```python
from build123d import *

# Parameters (mm, degrees)
IZIM1_R                     = 5
Y_KSEKLIK_EKSTR_ZYON1_DEPTH = 15
IZIM2_R                     = 7.5
Y_KSEKLIK_EKSTR_ZYON2_DEPTH = 5
RADYUS1_R                   = 5
Y_KSEKLIK_EKSTR_ZYON3_START = 5
IZIM3_R                     = 7.5
Y_KSEKLIK_EKSTR_ZYON3_DEPTH = 5
RADYUS2_R                   = 5


with BuildPart() as part:
    # Çizim1 → Yükseklik-Ekstrüzyon1 (new body)
    with BuildSketch(Plane.XY):
        Circle(IZIM1_R)
    extrude(amount=Y_KSEKLIK_EKSTR_ZYON1_DEPTH)

    # Çizim2 → Yükseklik-Ekstrüzyon2 (add)
    with BuildSketch(Plane.XY.offset(15)):
        Circle(IZIM2_R)
    extrude(amount=Y_KSEKLIK_EKSTR_ZYON2_DEPTH)

    # Radyus1
    radyus1_edges = [part.edges().sort_by_distance(p)[0] for p in [
        (-7.5, 0, 20),
    ]]
    fillet(radyus1_edges, radius=RADYUS1_R - 0.0001)  # a hair under: the kernel refuses the full size

    # Çizim3 → Yükseklik-Ekstrüzyon3 (add)
    with BuildSketch(Plane(origin=(0, 0, 0), x_dir=(-1, 0, 0), z_dir=(0, 0, -1)).offset(Y_KSEKLIK_EKSTR_ZYON3_START)):
        Circle(IZIM3_R)
    extrude(amount=-Y_KSEKLIK_EKSTR_ZYON3_DEPTH)

    # Radyus2
    radyus2_edges = [part.edges().sort_by_distance(p)[0] for p in [
        (7.5, 0, -5),
    ]]
    fillet(radyus2_edges, radius=RADYUS2_R - 0.0001)  # a hair under: the kernel refuses the full size


solid = part.part
```
The listing builds one solid part. Answer for the finished solid, in the listing's coordinates (mm). Give positions to 0.01 mm unless a question says otherwise; leave off trailing zeros. Order: outer loops, then holes, each group sorted by start corner. A loop starts at its lowest first (then second) coordinate and runs counter-clockwise, first axis right, second up.
Item 1: For a pull along Z with two mould halves and no side action, classify faces 1 (the face through (0, 0, 20)), 2 (the face through (0, 0, -5)), 3 (the face through (2, -5, 15)), 4 (the face through (-2, -5, 0)) as pulls with the +Z half, pulls with the -Z half, needs draft (parallel to the pull), parting line crosses it, or undercut.
From the geometry:
face 1: pulls with the +Z half
face 2: pulls with the -Z half
face 3: undercut
face 4: undercut
Item 2: Given pin 1 Ø2 at (y, z) = (-0.5, 5) entering from -X; pin 2 Ø3 at (x, z) = (-5.5, 6) entering from +Y; pin 3 Ø3 at (x, z) = (2, 2.5) entering from +Y, each flat-ended and moving along its own axis, determine where each tip first touches the part or whether it passes through.
From the geometry:
pin 1: stops at x = -5
pin 2: stops at y = 3
pin 3: stops at y = 4.97
Item 3: The part is cut by section A-A, the plane z = 11.75. Give the vertices of the cut face in (x, y), and give its area (3 significant figures).
From the geometry:
outline: circle Ø10 at (0, 0)
area: 78.5 mm2
Item 4: Find the intervals of material crossed by probe 1 along Z at (x, y) = (0, 5.25); probe 2 along Z at (x, y) = (5.5, 0.25); probe 3 along X at (y, z) = (0.25, -2.5), in increasing order.
From the geometry:
probe 1: z = -4.18 to 0, 15 to 19.18
probe 2: z = -4 to 0, 15 to 19
probe 3: x = -6.83 to 6.83
